```python
from build123d import *

# Parameters (mm, degrees)
SKETCH1_W           = 30
SKETCH1_H           = 30
BOSS_EXTRUDE1_DEPTH = 135
SKETCH2_W           = 20
SKETCH2_H           = 20
BOSS_EXTRUDE2_DEPTH = 10
SKETCH3_W           = 20.5
SKETCH3_H           = 20.5
CUT_EXTRUDE1_DEPTH  = 15
SKETCH4_W           = 20.5
SKETCH4_H           = 20.5
CUT_EXTRUDE2_DEPTH  = 15


with BuildPart() as part:
    # Sketch1 → Boss-Extrude1 (new body)
    with BuildSketch(Plane.XY):
        Rectangle(SKETCH1_W, SKETCH1_H)
    extrude(amount=BOSS_EXTRUDE1_DEPTH)

    # Sketch2 → Boss-Extrude2 (add)
    with BuildSketch(Plane.XY):
        Rectangle(SKETCH2_W, SKETCH2_H)
    extrude(amount=-BOSS_EXTRUDE2_DEPTH)

    # Sketch3 → Cut-Extrude1 (cut)
    with BuildSketch(Plane(origin=(15, 0, 0), x_dir=(0, 0, -1), z_dir=(1, 0, 0))):
        with Locations((-120, 0)):
            Rectangle(SKETCH3_W, SKETCH3_H)
    extrude(amount=-CUT_EXTRUDE1_DEPTH, mode=Mode.SUBTRACT)

    # Sketch4 → Cut-Extrude2 (cut)
    with BuildSketch(Plane(origin=(0, 15, 0), x_dir=(1, 0, 0), z_dir=(0, 1, 0))):
        with Locations((0, -120)):
            Rectangle(SKETCH4_W, SKETCH4_H)
    extrude(amount=-CUT_EXTRUDE2_DEPTH, mode=Mode.SUBTRACT)


solid = part.part
```
Read the model definition and answer for the solid it produces. Units are mm, in the model's axes. A direction names the side the tool comes from. Coordinates: 2 decimals unless noted, no trailing zeros. Order: outer loops, then holes, each group sorted by start corner. A loop starts at its lowest first (then second) coordinate and runs counter-clockwise, first axis right, second up. Notation, with made-up numbers: (-20, -40) - (28, -40) arc R20 ccw to (28, -22) - close; hole circle Ø4 at (-18, -37). An arc over 180 degrees is marked (long way). Answer as a JSON object with one key per item and string values. Group by question number.
Item 1: Section B-B (y = 2.75) is taken. Give the vertices of the cut face in (x, z).
Item 2: Section A-A (z = 119.5) is taken. Give the vertices of the cut face in (x, y), plus the area to 3 significant figures.
Item 3: A tool of negligible diameter and unlimited length cuts with its end or side. For faces 1 (the face through (0, -5, 120)), 2 (the face through (-10, 0, -5)), 3 (the face through (0, 10, -5)), 4 (the face through (8, -10.25, 120)), 5 (the face through (10, 0, -5)), from which of +Z, -Z, +X, -X, +Y, -Y can it reach the whole face along a straight path? Write none if from no direction.
Item 4: Flat-ended cylindrical pins translate along their axes: P1, Ø4.5, axis at x = 6.5, z = 116.5, coming from the +Y side; P2, Ø11, axis at x = -1.5, z = -7, coming from the -Y side; P3, Ø3, axis at y = -6, z = 119.5, coming from the +X side. Find the tip coordinate at first contact, or state that the pin passes through.
Item 5: Consider probe 1 along Z at (x, y) = (7.75, -8.75); probe 2 along Z at (x, y) = (-5, 10.5); probe 3 along Y at (x, z) = (8.5, 120). Determine where each line is inside the solid, lowest interval first. Write a range as from..to.
Item 6: Section C-C (x = -6.75) is taken. Give the vertices of the cut face in (y, z).
Item 7: Section D-D (y = -11.5) is taken. Give the vertices of the cut face in (x, z), plus the area to 3 significant figures.
Item 8: The mould has two halves that part along Y. Classify faces 6 (the face through (15, 0, 52)), 7 (the face through (0, -15, 67)), 8 (the face through (-5, 0, 120)), 9 (the face through (13, 10.25, 120)): +Y half, -Y half, draft (parallel to the pull), parting line (faces both ways), or undercut.
Results are:
{
 "1": {"outline": "(-15, 0) - (-10, 0) - (-10, -10) - (10, -10) - (10, 0) - (15, 0) - (15, 109.75) - (-10.25, 109.75) - (-10.25, 130.25) - (15, 130.25) - (15, 135) - (-15, 135) - close"},
 "2": {"outline": "(-15, -15) - (15, -15) - (15, -10.25) - (0, -10.25) - (0, 0) - (-10.25, 0) - (-10.25, 15) - (-15, 15) - close; (10.25, 10.25) - (15, 10.25) - (15, 15) - (10.25, 15) - close", "area": "390 mm^2"},
 "3": {"face 1": "+X, +Y", "face 2": "-Z, -X, +Y, -Y", "face 3": "-Z, +X, -X, +Y", "face 4": "+X", "face 5": "-Z, +X, +Y, -Y"},
 "4": {"P1": "stops at y = -10.25", "P2": "stops at y = -10", "P3": "stops at x = 0"},
 "5": {"probe 1": "z = -10..109.75, 130.25..135", "probe 2": "z = 0..109.75, 130.25..135", "probe 3": "y = -15..-10.25"},
 "6": {"outline": "(-15, 0) - (-10, 0) - (-10, -10) - (10, -10) - (10, 0) - (15, 0) - (15, 109.75) - (0, 109.75) - (0, 130.25) - (15, 130.25) - (15, 135) - (-15, 135) - close"},
 "7": {"outline": "(-15, 0) - (15, 0) - (15, 135) - (-15, 135) - close", "area": "4,050 mm^2"},
 "8": {"face 6": "draft", "face 7": "-Y half", "face 8": "+Y half", "face 9": "undercut"}
}
